Autodesk Fusion 360 part; units mm, degrees
sketch "Sketch1" plane through (0, 0, 0) normal (0, 0, 1) x (1, 0, 0)
  line L0 (0, 0) -> (6, 0)
  line L1 (6, 0) -> (6, 6)
  line L2 (6, 6) -> (0, 6)
  line L3 (0, 6) -> (0, 0)
  line L4 (6, 0) -> (8, 0)
  line L5 (8, 0) -> (8, 30)
  line L6 (8, 30) -> (6, 30)
  line L7 (6, 30) -> (6, 0)
  line L8 (6, 30) -> (25, 30)
  line L9 (25, 30) -> (25, 28)
  line L10 (25, 28) -> (6, 28)
  line L11 (6, 28) -> (6, 30)
  line L12 (50, 6) -> (50, 0)
  line L13 (44, 6) -> (50, 6)
  line L14 (44, 0) -> (42, 0)
  line L15 (50, 0) -> (44, 0)
  line L16 (44, 30) -> (25, 30)
  line L17 (42, 0) -> (42, 30)
  line L18 (44, 0) -> (44, 6)
  line L19 (44, 30) -> (44, 0)
  line L20 (25, 28) -> (44, 28)
  line L21 (44, 28) -> (44, 30)
  line L22 (42, 30) -> (44, 30)
  point P0 (50, 0)
  dimension "d1" = 6
  dimension "d2" = 6
  dimension "d3" = 2
  dimension "d4" = 30
  dimension "d5" = 19
  dimension "d6" = 2
extrude "Extrude1" add sketch "Sketch1" along normal blind 3 and the other way blind 3 contours L0 L1 L2 L3 L7 | L12 L13 L15 L18 L19 makes body 1 at (0, 2, 1) makes body 2 at (46, 2, 3)
extrude "Extrude2" add sketch "Sketch1" along normal blind 1.5 and the other way blind 1.5 contours L1 L4 L5 L7 L10 | L5 L6 L7 L8 L10 L11 | L5 L8 L9 L10 | L9 L16 L17 L20 | L14 L17 L18 L19 L20 | L16 L17 L19 L20 L21 L22 bodies 1 2
sketch "Sketch2" plane through (0, 6, 0) normal (0, 1, 0) x (-1, 0, 0)
  line L0 (0, -3) -> (0, 3)
  line L1 (0, 3) -> (-6, 3)
  line L2 (-6, 3) -> (-6, 1.5)
  line L3 (-6, 1.5) -> (-6, -1.5)
  line L4 (-6, -1.5) -> (-6, -3)
  line L5 (-6, -3) -> (0, -3)
  circle A0 centre (-3, 0) radius 1.5
  circle A1 centre (-47, 0) radius 1.5
  line L6 (-50, -3) -> (-50, 3)
  line L7 (-44, -3) -> (-50, -3)
  dimension "d15" = 3
  dimension "d16" = 3
  dimension "d17" = 3
  dimension "d18" = 3
  dimension "d19" = 3
  dimension "d20" = 3
extrude "Extrude3" cut sketch "Sketch2" against normal blind 18 contours A0 | A1 bodies 1
extrude "Extrude4" add 1 faces at (7.3333, 11.3333, 1.5) along direction (0, 0, 1) blind 1.5 on bodies 1 bodies 1
Could you check a few things on this model? Use its own coordinates, in mm. A direction names the side the tool comes from. Round coordinates to 2 decimals unless told otherwise and drop trailing zeros. Loops run counter-clockwise (first coordinate to the right, second up) from the corner with the lowest first, then second, coordinate; pieces in that order, holes last. Notation, with made-up numbers: (81.5, 20) - (92.5, 20) arc R21 cw to (92.5, 52) - close; hole circle Ø4 at (57, -3.75). An arc over 180 degrees is marked (long way). Answer in a Markdown table with one row per item. Add a question column.
(1) If we mould it in two halves opening along Z, with no side actions, what happens to faces 1 (the face through (47, 3, -3)), 2 (the face through (6, 3, -2)), 3 (the face through (48.5, 3.04, 0.07))? For each: pulls with the +Z half, pulls with the -Z half, needs draft (parallel to the pull), parting line crosses it, or undercut.
(2) I'm going to push flat-ended pins straight in: pin 1 (6 mm diameter, centred on x = 10.5, y = 6, fed in from -Z); pin 2 (1.5 mm diameter, centred on x = 32, z = 0.5, fed in from -Y); pin 3 (3.5 mm diameter, centred on y = 21.5, z = 0.5, fed in from -X); pin 4 (15 mm diameter, centred on x = 20, y = 14, fed in from -Z). Where does each tip first touch, or does it pass through?
(3) If we section it at A-A (y = 17.5): Please give me the cut outline in (x, z), plus the area to 3 significant figures.
(4) I need wall thicknesses on line 1 along Z through (x, y) = (47, 2.3); line 2 along X through (y, z) = (12.25, 0.5); line 3 along X through (y, z) = (2.25, -0.9). Which ranges of each line are inside material? Lowest first, please.
(5) If we section it at B-B (z = -2.05): Please give me the cut outline in (x, y), plus the area to 3 significant figures.
(6) For faces 4 (the face through (25, 28, 1)), 5 (the face through (4.4, 6, -1.4)), 6 (the face through (44, 3, -2)), which set-ups out of +Z, -Z, +X, -X, +Y, -Y let a thin tool reach every point of the face, with its end or its side?
(7) If we section it at C-C (x = 39.5): Please give me the cut outline in (y, z), plus the area to 3 significant figures.
Model answer:
| question | item | result |
|---|---|---|
| 1 | face 1 | pulls with the -Z half |
| 1 | face 2 | needs draft |
| 1 | face 3 | undercut |
| 2 | pin 1 | stops at z = -1.5 |
| 2 | pin 2 | stops at y = 28 |
| 2 | pin 3 | stops at x = 6 |
| 2 | pin 4 | passes through |
| 3 | outline | (6, -1.5) - (8, -1.5) - (8, 3) - (6, 3) - close; (42, -1.5) - (44, -1.5) - (44, 3) - (42, 3) - close |
| 3 | area | 18.0 mm² |
| 4 | line 1 | z = -3 to -1.5, 1.5 to 3 |
| 4 | line 2 | x = 6 to 8, 42 to 44 |
| 4 | line 3 | x = 0 to 1.8, 4.2 to 8, 42 to 45.8, 48.2 to 50 |
| 5 | outline | (0, 0) - (6, 0) - (6, 6) - (0, 6) - close; (44, 0) - (50, 0) - (50, 6) - (44, 6) - close |
| 5 | area | 72.0 mm² |
| 6 | face 4 | +Z, -Z, -Y |
| 6 | face 5 | +Z, -Z, -X, +Y |
| 6 | face 6 | -Z, +Y, -Y |
| 7 | outline | (28, -1.5) - (30, -1.5) - (30, 3) - (28, 3) - close |
| 7 | area | 9.00 mm² |
